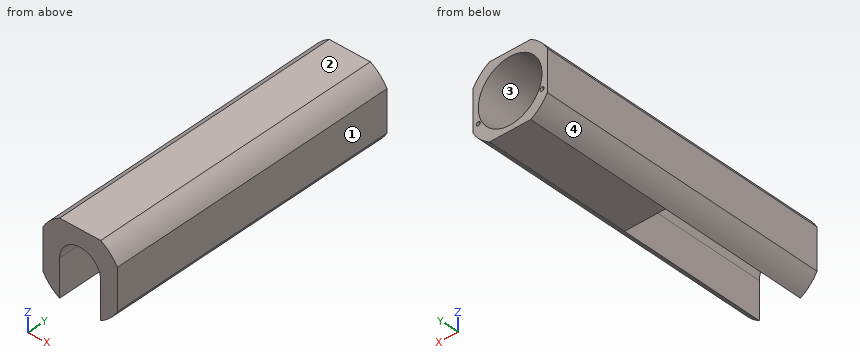
```python
from build123d import *

# Parameters (mm, degrees)
F0_R     = 2.38125
F0_R_2   = 38.1
F1_DEPTH = 165.1
F2_R     = 19.05
F3_DEPTH = 12.7
F5_DEPTH = 177.8


with BuildPart() as f1:
    # F0 (on Front) → F1 (new body)
    with BuildSketch(Plane.XZ):
        with BuildLine():
            Line((24.593444, 44.45), (-24.593444, 44.45))
            ThreePointArc((-24.593444, 44.45), (-35.921024, 35.921024), (-44.45, 24.593444))
            Line((-44.45, 24.593444), (-44.45, -24.593444))
            ThreePointArc((-44.45, -24.593444), (-35.921024, -35.921024), (-24.593444, -44.45))
            Line((-24.593444, -44.45), (24.593444, -44.45))
            ThreePointArc((24.593444, -44.45), (35.921024, -35.921024), (44.45, -24.593444))
            Line((44.45, -24.593444), (44.45, 24.593444))
            ThreePointArc((44.45, 24.593444), (35.921024, 35.921024), (24.593444, 44.45))
        make_face()
        with Locations((-38.1, -17.4625)):
            Circle(F0_R, mode=Mode.SUBTRACT)
        with Locations((38.1, -17.4625)):
            Circle(F0_R, mode=Mode.SUBTRACT)
        Circle(F0_R_2, mode=Mode.SUBTRACT)
    extrude(amount=F1_DEPTH)

    # F2 (on face) → F3 (join)
    with BuildSketch(Plane.XZ.offset(165.1)):
        with BuildLine():
            Line((24.593444, 44.45), (-24.593444, 44.45))
            ThreePointArc((-24.593444, 44.45), (-35.921024, 35.921024), (-44.45, 24.593444))
            Line((-44.45, 24.593444), (-44.45, -24.593444))
            ThreePointArc((-44.45, -24.593444), (-35.921024, -35.921024), (-24.593444, -44.45))
            Line((-24.593444, -44.45), (24.593444, -44.45))
            ThreePointArc((24.593444, -44.45), (35.921024, -35.921024), (44.45, -24.593444))
            Line((44.45, -24.593444), (44.45, 24.593444))
            ThreePointArc((44.45, 24.593444), (35.921024, 35.921024), (24.593444, 44.45))
        make_face()
        Circle(F2_R, mode=Mode.SUBTRACT)
    extrude(amount=F3_DEPTH)

    # F4 (on face) → F5 (join)
    with BuildSketch(Plane.XZ.offset(177.8)):
        with BuildLine():
            Line((24.593444, 44.45), (-24.593444, 44.45))
            ThreePointArc((-24.593444, 44.45), (-35.921024, 35.921024), (-44.45, 24.593444))
            Line((-44.45, 24.593444), (-44.45, -24.593444))
            ThreePointArc((-44.45, -24.593444), (-35.921024, -35.921024), (-24.593444, -44.45))
            Line((-24.593444, -44.45), (-24.5872, 0))
            ThreePointArc((-24.5872, 0), (0, 24.5872), (24.5872, 0))
            Line((24.5872, 0), (24.593444, -44.45))
            ThreePointArc((24.593444, -44.45), (35.921024, -35.921024), (44.45, -24.593444))
            Line((44.45, -24.593444), (44.45, 24.593444))
            ThreePointArc((44.45, 24.593444), (35.921024, 35.921024), (24.593444, 44.45))
        make_face()
    extrude(amount=F5_DEPTH)


solid = f1.part
```
Geometry: final body of the model. Coordinates: model frame, mm. Face numbers are marked on the shaded views. Round coordinates to 2 decimals unless told otherwise and drop trailing zeros. Write each loop counter-clockwise with the first axis right and the second up, starting at its lowest first coordinate (ties: lowest second). Pieces come first, ordered by that corner, then holes. Notation, with made-up numbers: M 31.25,72 L 85.25,72 A16 ccw 85.25,78 Z; hole C 1.5,-5.75 d1. An arc over 180 degrees is marked long. Answer in a Markdown table with one row per item. Add a question column.
(1) Cut plane B-B, the plane y = -300. Return the cut outline in (x, z), then the cut area to 3 significant figures.
(2) Draft query along Z for the marked faces 1, 2, 3 and 4. Return one class per face: pulls with the +Z half, pulls with the -Z half, needs draft (parallel to the pull), parting line crosses it, or undercut.
(3) Cut plane C-C, the plane z = 34. Return the cut outline in (x, y), then the cut area to 3 significant figures.
(4) Cut plane A-A, the plane x = 0. Return the cut outline in (y, z).
(5) Contact query for flat-ended pins moving along their axis: pin 1 (5 mm diameter, centred on x = 37.5, z = -17.5, fed in from +Y); pin 2 (5 mm diameter, centred on x = 10.5, z = -30.5, fed in from -Y); pin 3 (4 mm diameter, centred on x = 11.5, z = -17, fed in from +Y). Output: stop coordinate, or through.
(6) Ray query, L1, parallel to Z at x = 0, y = -78; L2, parallel to X at y = -299, z = -18.5; L3, parallel to Y at x = 30, z = 23. Return the intervals inside material, ascending.
(7) Cut plane D-D, the plane y = -23. Return the cut outline in (x, z).
Established:
| question | item | result |
|---|---|---|
| 1 | outline | M -44.45,-24.59 A50.8 ccw -24.59,-44.45 L -24.59,0 A24.59 cw 24.59,0 L 24.59,-44.45 A50.8 ccw 44.45,-24.59 L 44.45,24.59 A50.8 ccw 24.59,44.45 L -24.59,44.45 A50.8 ccw -44.45,24.59 Z |
| 1 | area | 4,130 mm² |
| 2 | face 1 | needs draft |
| 2 | face 2 | pulls with the +Z half |
| 2 | face 3 | undercut |
| 2 | face 4 | pulls with the -Z half |
| 3 | outline | M -37.74,-355.6 L 37.74,-355.6 L 37.74,0 L 17.19,0 L 17.19,-165.1 L -17.19,-165.1 L -17.19,0 L -37.74,0 Z |
| 3 | area | 21,200 mm² |
| 4 | outline | M -355.6,24.59 L -177.8,24.59 L -177.8,19.05 L -165.1,19.05 L -165.1,38.1 L 0,38.1 L 0,44.45 L -355.6,44.45 Z; M -177.8,-44.45 L 0,-44.45 L 0,-38.1 L -165.1,-38.1 L -165.1,-19.05 L -177.8,-19.05 Z |
| 5 | pin 1 | y = 0 |
| 5 | pin 2 | y = -177.8 |
| 5 | pin 3 | y = -165.1 |
| 6 | L1 | -44.45 to -38.1, 38.1 to 44.45 |
| 6 | L2 | -44.45 to -24.59, 24.59 to 44.45 |
| 6 | L3 | -355.6 to -165.1 |
| 7 | outline | M -44.45,-24.59 A50.8 ccw -24.59,-44.45 L 24.59,-44.45 A50.8 ccw 44.45,-24.59 L 44.45,24.59 A50.8 ccw 24.59,44.45 L -24.59,44.45 A50.8 ccw -44.45,24.59 Z; hole C -38.1,-17.46 d4.76; hole C 0,0 d76.2; hole C 38.1,-17.46 d4.76 |
